The model under review builds one solid part; all positions refer to its coordinate system, in mm. A direction names the side the tool comes from. Coordinates: 2 decimals unless noted, no trailing zeros. Loops run counter-clockwise (first coordinate to the right, second up) from the corner with the lowest first, then second, coordinate; pieces in that order, holes last. Notation, with made-up numbers: M 15,45.25 L 32,45.25 A14 ccw 32,61.25 Z; hole C -23.75,35 d3. An arc over 180 degrees is marked long. Write item = value, one per line. Start each with the question number.
Q1. We need section C-C on z = -0.65. Give the boundary of the cut face in (x, y) (1 decimal), and give its area (3 significant figures).
Q2. For faces 5 (the face through (117, -34, -2.6)), 6 (the face through (118.95, -35.12, -1.28)), list the 3-axis set-ups (+Z, -Z, +X, -X, +Y, -Y) from which the entire face can be reached by the end or side of a thin tool; tool diameter is ignored.
Q3. We need section D-D on y = -21.5. Give the boundary of the cut face in (x, z), and give its area (3 significant figures).
Q4. Wall thickness on probe 1 along Z at (x, y) = (97.75, -32); probe 2 along X at (y, z) = (-27, -2.7); probe 3 along Y at (x, z) = (95, -2.65): over which ranges is each line inside the solid? List them lowest first.
Q5. We need section B-B on y = -36. Give the boundary of the cut face in (x, z).
Q6. We need section A-A on x = 116.75. Give the boundary of the cut face in (y, z), and give its area (3 significant figures).
Q7. Clearance check with flat-ended pins moving along their axes: pin 1 Ø4 at (x, y) = (97.59, -29.1) entering from +Z; pin 2 Ø1.5 at (x, z) = (105, -2.5) entering from +Y; pin 3 Ø5 at (x, y) = (97.59, -29.1) entering from -Z. State where each tip first meets the part, or that it passes through.
Q8. Mouldability with a two-part tool opening along Y and no side actions: class faces 1 (the face through (113.3, -18.5, -1.3)), 2 (the face through (102.04, -20.45, -1.48)), 3 (the face through (97.269, -30.565, -1.282)), 4 (the face through (111, -27, 0)) as released by +Y, released by -Y, zero draft, split by the parting line, or undercut.
Autodesk Inventor part; units mm, degrees
ref_plane "YZ Plane" through (0, 0, 0) normal (1, 0, 0) x (0, 1, 0)
ref_plane "XZ Plane" through (0, 0, 0) normal (0, 1, 0) x (-1, 0, 0)
ref_plane "XY Plane" through (0, 0, 0) normal (0, 0, 1) x (1, 0, 0)
sketch "スケッチ1" plane through (0, 0, 0) normal (0, 0, 1) x (1, 0, 0)
  circle A0 centre (117.5177, -35.5687) radius 1.5
  circle A1 centre (95.4507, -12.9865) radius 1.5
  circle A2 centre (97.5945, -29.101) radius 1.5
  circle A3 centre (111.885, -19) radius 1.5
  line L0 (116.6369, -13.86) -> (104.8897, -3)
  line L1 (104.8897, -3) -> (101.885, -3)
  arc A4 (99.885, -3) -> (101.885, -3) centre (100.885, -3) ccw
  line L2 (99.885, -3) -> (99.885, 0)
  line L3 (99.885, 0) -> (84.885, 0)
  line L4 (84.885, 0) -> (84.885, -3)
  arc A5 (82.885, -3) -> (84.885, -3) centre (83.885, -3) ccw
  line L5 (82.885, -3) -> (81.4397, -3)
  arc A6 (79.4397, -3) -> (81.4397, -3) centre (80.4397, -3) ccw
  line L6 (79.4397, -3) -> (79.4397, 0)
  line L7 (79.4397, 0) -> (64.4397, 0)
  line L8 (64.4397, 0) -> (64.4397, -3)
  arc A7 (62.4397, -3) -> (64.4397, -3) centre (63.4397, -3) ccw
  line L9 (62.4397, -3) -> (59.4397, -3)
  line L10 (59.4397, -3) -> (59.4397, -6)
  line L11 (59.4397, -6) -> (65.1115, -8.2188)
  arc A8 (65.1115, -8.2188) -> (69.3788, -9.8882) centre (68.4397, -6) ccw
  line L12 (69.3788, -9.8882) -> (97.5091, -20.8927)
  arc A9 (97.5091, -20.8927) -> (98.5543, -24.7045) centre (111.885, -19) ccw
  arc A10 (98.5543, -24.7045) -> (97.6262, -33.6009) centre (97.5945, -29.101) ccw
  line L13 (97.6262, -33.6009) -> (107.1669, -33.5336)
  line L14 (107.1669, -33.5336) -> (114.849, -39.192)
  arc A11 (114.849, -39.192) -> (121.9415, -34.7438) centre (117.5177, -35.5687) ccw
  line L15 (121.9415, -34.7438) -> (118.7664, -17.7168)
  arc A12 (118.7664, -17.7168) -> (116.6369, -13.86) centre (111.885, -19) ccw
  line L16 (69.4397, -3) -> (74.4397, -3)
  arc A13 (76.4397, -3) -> (74.4397, -3) centre (75.4397, -3) ccw
  line L17 (76.4397, -3) -> (76.4397, -6)
  arc A14 (74.4397, -6) -> (76.4397, -6) centre (75.4397, -6) ccw
  line L18 (74.4397, -6) -> (69.4397, -6)
  arc A15 (67.4397, -6) -> (69.4397, -6) centre (68.4397, -6) ccw
  line L19 (67.4397, -6) -> (67.4397, -3)
  arc A16 (69.4397, -3) -> (67.4397, -3) centre (68.4397, -3) ccw
  arc A17 (94.885, -6) -> (96.885, -6) centre (95.885, -6) ccw
  line L20 (94.885, -6) -> (89.885, -6)
  arc A18 (87.885, -6) -> (89.885, -6) centre (88.885, -6) ccw
  line L21 (87.885, -6) -> (87.885, -3)
  arc A19 (89.885, -3) -> (87.885, -3) centre (88.885, -3) ccw
  line L22 (89.885, -3) -> (94.885, -3)
  arc A20 (96.885, -3) -> (94.885, -3) centre (95.885, -3) ccw
  line L23 (96.885, -3) -> (96.885, -6)
  circle A21 centre (97.5945, -29.101) radius 4.5
  circle A22 centre (111.885, -19) radius 4.5
  circle A23 centre (117.5177, -35.5687) radius 4.5
  line L24 (94.9971, -25.4263) -> (109.2877, -15.3253)
  line L25 (116.1456, -17.5516) -> (121.7783, -34.1203)
  line L26 (116.1283, -39.8488) -> (96.205, -33.3811)
  point P0 (0, 0)
  point P1 (0, 0)
  dimension "d0" = 9
extrude "押し出し1" add sketch "スケッチ1" against normal blind 3 contours A11 A23 | A23 L14 L13 A21 A9 L24 A22 L25 | L26 A10 L13 L14 A11 | A22 | A10 A21 | L24 A9 A10
sketch "スケッチ2" plane through (0, 0, -3) normal (0, 0, -1) x (-1, 0, 0)
  line L0 (-94.9971, -25.4263) -> (-109.2877, -15.3253)
  arc A0 (-109.2877, -15.3253) -> (-116.1456, -17.5516) centre (-111.885, -19) ccw
  line L1 (-116.1456, -17.5516) -> (-121.7783, -34.1203)
  arc A1 (-121.7783, -34.1203) -> (-116.1283, -39.8488) centre (-117.5177, -35.5687) ccw
  line L2 (-116.1283, -39.8488) -> (-96.205, -33.3811)
  arc A2 (-96.205, -33.3811) -> (-94.9971, -25.4263) centre (-97.5945, -29.101) ccw
  circle A3 centre (-111.885, -19) radius 1.5
  circle A4 centre (-97.5945, -29.101) radius 1.5
  circle A5 centre (-117.5177, -35.5687) radius 1.5
  circle A6 centre (-97.5945, -29.101) radius 1.5
  circle A7 centre (-97.5945, -29.101) radius 3
  circle A8 centre (-111.885, -19) radius 1.5
  circle A9 centre (-111.885, -19) radius 3
  circle A10 centre (-117.5177, -35.5687) radius 1.5
  circle A11 centre (-117.5177, -35.5687) radius 3
  point P0 (0, 0)
  dimension "d3" = 6
  dimension "d4" = 6
  dimension "d6" = 6
extrude "押し出し2" cut sketch "スケッチ2" against normal blind 0.4 contours A5 | A7 | A9 | A11
properties part number "後ろウィング固定フレーム押さえ"
Returned:
q1.outline = M 95,-25.4 A4.5 ccw 96.2,-33.4 L 116.1,-39.8 A4.5 ccw 121.9,-34.7 A4.5 ccw 121.8,-34.1 L 116.1,-17.6 A4.5 ccw 109.3,-15.3 Z; hole C 97.6,-29.1 d3; hole C 111.9,-19 d3; hole C 117.5,-35.6 d3
q1.area = 441 mm^2
q2.face_5 = -Z
q2.face_6 = +Z, -Z
q3.outline = M 100.55,-3 L 110.23,-3 L 110.23,-2.6 L 113.54,-2.6 L 113.54,-3 L 117.49,-3 L 117.49,0 L 100.55,0 Z
q3.area = 49.5 mm^2
q4.probe_1 = -2.6 to 0
q4.probe_2 = 93.62 to 95.45, 99.74 to 119.36
q4.probe_3 = -32.78 to -30.61, -27.59 to -25.42
q5.outline = M 104.27,-3 L 114.55,-3 L 114.55,-2.6 L 116.08,-2.6 L 116.08,0 L 104.27,0 Z; M 118.95,-2.6 L 120.49,-2.6 L 120.49,-3 L 122,-3 L 122,0 L 118.95,0 Z
q6.outline = M -40,-3 L -38.47,-3 L -38.47,-2.6 L -36.86,-2.6 L -36.86,0 L -40,0 Z; M -34.28,-2.6 L -32.67,-2.6 L -32.67,-3 L -19.33,-3 L -19.33,0 L -34.28,0 Z
q6.area = 53.0 mm^2
q7.pin_1 = 0
q7.pin_2 = -17.83
q7.pin_3 = -2.6
q8.face_1 = undercut
q8.face_2 = released by +Y
q8.face_3 = undercut
q8.face_4 = zero draft
